Answer from the drawing. Dimensions are ordinates in mm from the lowest x, y and z of the part. A direction names the side the tool comes from. Give positions to 0.01 mm unless a question says otherwise; leave off trailing zeros. Order: outer loops, then holes, each group sorted by start corner. A loop starts at its lowest first (then second) coordinate and runs counter-clockwise, first axis right, second up. Notation, with made-up numbers: M 29.25,27.25 L 80.25,27.25 A36 cw 80.25,64.25 Z; hole C 48.25,72.5 d5. An arc over 180 degrees is marked long. One line per item, written item: value.
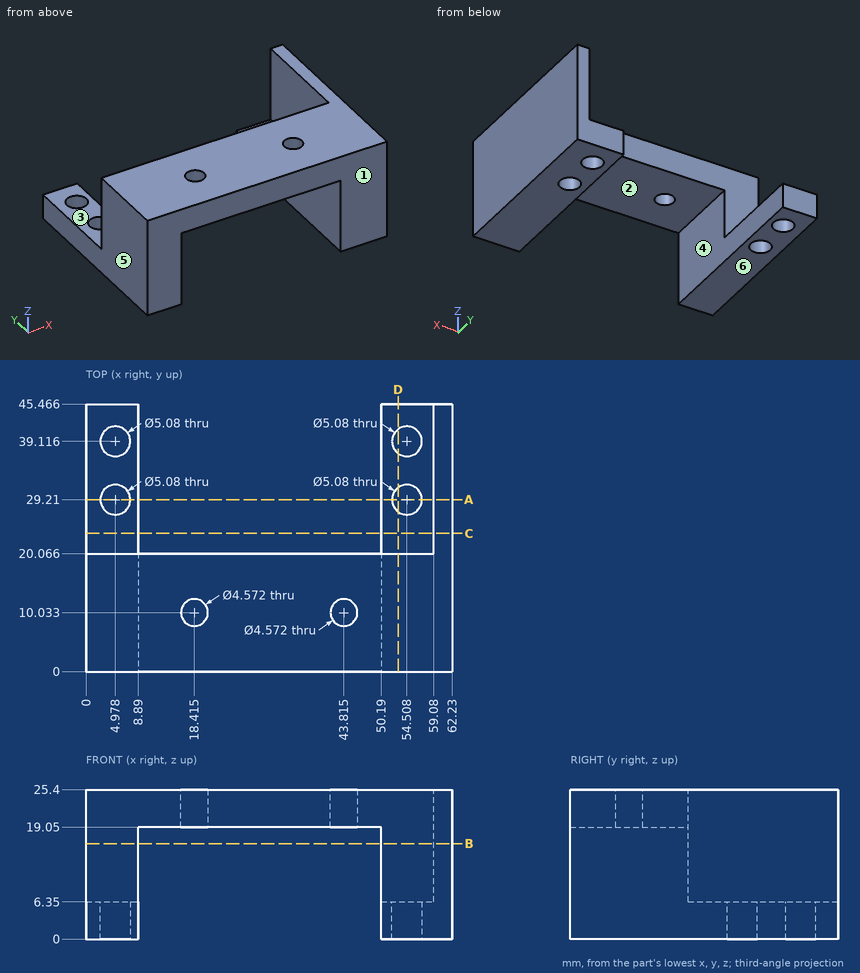
(1) Section D-D, the plane x = 53 is taken. Give the vertices of the cut face in (y, z), then the cut area to 3 significant figures.
Findings:
outline: M 0,0 L 27.17,0 L 27.17,6.35 L 20.07,6.35 L 20.07,25.4 L 0,25.4 Z; M 31.25,0 L 37.07,0 L 37.07,6.35 L 31.25,6.35 Z; M 41.16,0 L 45.47,0 L 45.47,6.35 L 41.16,6.35 Z
area: 619 mm^2
(2) Which of the six approach directions +Z, -Z, +X, -X, +Y, -Y give full straight-line access (tool end or side, diameter ignored) to the marked faces 1, 2 and 3?
Findings:
face 1: +Z, -Z, +X, -X, -Y
face 2: -Z, +Y, -Y
face 3: +Z, -X, +Y
(3) Determine the mould class of the marked faces 4, 5 and 6 for opening direction X: pulls with the +X half, pulls with the -X half, needs draft (parallel to the pull), parting line crosses it, or undercut.
Findings:
face 4: undercut
face 5: pulls with the -X half
face 6: needs draft
(4) Section B-B, the plane z = 16.25 is taken. Give the vertices of the cut face in (x, y).
Findings:
outline: M 0,0 L 8.89,0 L 8.89,20.07 L 0,20.07 Z; M 50.19,0 L 62.23,0 L 62.23,45.47 L 59.08,45.47 L 59.08,20.07 L 50.19,20.07 Z
(5) Section C-C, the plane y = 23.5 is taken. Give the vertices of the cut face in (x, z), then the cut area to 3 significant figures.
Findings:
outline: M 0,0 L 8.89,0 L 8.89,6.35 L 0,6.35 Z; M 50.19,0 L 62.23,0 L 62.23,25.4 L 59.08,25.4 L 59.08,6.35 L 50.19,6.35 Z
area: 193 mm^2
(6) Section A-A, the plane y = 29.21 is taken. Give the vertices of the cut face in (x, z).
Findings:
outline: M 0,0 L 2.44,0 L 2.44,6.35 L 0,6.35 Z; M 7.52,0 L 8.89,0 L 8.89,6.35 L 7.52,6.35 Z; M 50.19,0 L 51.97,0 L 51.97,6.35 L 50.19,6.35 Z; M 57.05,0 L 62.23,0 L 62.23,25.4 L 59.08,25.4 L 59.08,6.35 L 57.05,6.35 Z
(7) Find the intervals of material crossed by probe 1 along X at (y, z) = (43.5, 1.5); probe 2 along Z at (x, y) = (46.5, 11); probe 3 along Z at (x, y) = (57, 44), in increasing order. Write a range as from..to.
Findings:
probe 1: x = 0..8.89, 50.19..62.23
probe 2: z = 19.05..25.4
probe 3: z = 0..6.35
(8) Given P1, Ø2.5, axis at x = 3.5, y = 36.5, coming from the +Z side; P2, Ø9.5, axis at y = 28, z = 7, coming from the -X side; P3, Ø1.5, axis at x = 46.5, z = 19.5, coming from the +Y side; P4, Ø4, axis at y = 37.5, z = 22.5, coming from the -X side, each flat-ended and moving along its own axis, determine where each tip first touches the part or whether it passes through.
Findings:
P1: stops at z = 6.35
P2: stops at x = 0
P3: stops at y = 20.07
P4: stops at x = 59.08
